from build123d import *

# Parameters (mm, degrees)
BOSS_EXTRUDE1_DEPTH       = 4.7625
SKETCH2_R                 = 3.302
BOSS_EXTRUDE2_DEPTH       = 3.175
SKETCH3_W                 = 12.827
SKETCH3_H                 = 4.8768
SKETCH3_W_2               = 4.8768
SKETCH3_H_2               = 12.827
PANEL_SLOTS_DEPTH         = 5.7625
BOSS_EXTRUDE8_DEPTH       = 4.7625
F_6_CLEARANCE_HOLE2_D     = 3.7973
F_6_CLEARANCE_HOLE2_DEPTH = 25.4
F_6_CLEARANCE_HOLE2_TIP   = 1.140824014
BOSS_EXTRUDE9_DEPTH       = 4.7625
F_6_CLEARANCE_HOLE3_D     = 3.7973
F_6_CLEARANCE_HOLE3_DEPTH = 25.4
F_6_CLEARANCE_HOLE3_TIP   = 1.140824014
FILLET1_R                 = 2.54
FILLET2_R                 = 2.54


with BuildPart() as part:
    # Sketch1 → Boss-Extrude1 (new body)
    with BuildSketch(Plane.XY):
        Polygon((-150.669615327, -62.417005507), (-62.404018861, -150.674994572), (62.417005507, -150.669615327), (150.674994572, -62.404018861), (150.669615327, 62.417005507), (62.404018861, 150.674994572), (-62.417005507, 150.669615327), (-150.674994572, 62.404018861), align=None)
        Polygon((-137.969842044, -57.155945955), (-57.144053939, -137.974767879), (57.155945955, -137.969842044), (137.974767879, -57.144053939), (137.969842044, 57.155945955), (57.144053939, 137.974767879), (-57.155945955, 137.969842044), (-137.974767879, 57.144053939), align=None, mode=Mode.SUBTRACT)
    extrude(amount=BOSS_EXTRUDE1_DEPTH)

    # Sketch2 → Boss-Extrude2 (add)
    with BuildSketch(Plane.XY.offset(4.7625)):
        with BuildLine():
            Line((-104.300258744, 90.821465649), (-90.83045509, 104.292430334))
            ThreePointArc((-90.83045509, 104.292430334), (-90.829874575, 90.822046164), (-104.300258744, 90.821465649))
        make_face()
        with Locations((-94.197615746, 94.189497078)):
            Circle(SKETCH2_R, mode=Mode.SUBTRACT)
        with BuildLine():
            Line((104.292430334, 90.83045509), (90.821465649, 104.300258744))
            ThreePointArc((90.821465649, 104.300258744), (90.822046164, 90.829874575), (104.292430334, 90.83045509))
        make_face()
        with Locations((94.189497078, 94.197615746)):
            Circle(SKETCH2_R, mode=Mode.SUBTRACT)
        with BuildLine():
            Line((104.300258744, -90.821465649), (90.83045509, -104.292430334))
            ThreePointArc((90.83045509, -104.292430334), (90.829874575, -90.822046164), (104.300258744, -90.821465649))
        make_face()
        with Locations((94.197615746, -94.189497078)):
            Circle(SKETCH2_R, mode=Mode.SUBTRACT)
        with BuildLine():
            Line((-104.292430334, -90.83045509), (-90.821465649, -104.300258744))
            ThreePointArc((-90.821465649, -104.300258744), (-90.822046164, -90.829874575), (-104.292430334, -90.83045509))
        make_face()
        with Locations((-94.189497078, -94.197615746)):
            Circle(SKETCH2_R, mode=Mode.SUBTRACT)
    extrude(amount=-BOSS_EXTRUDE2_DEPTH)

    # Sketch3 → Panel Slots (cut, through all)
    with BuildSketch(Plane.XY.offset(4.7625)):
        with Locations((-38.105945973, 145.908163017)):
            Rectangle(SKETCH3_W, SKETCH3_H)
        with Locations((12.69405398, 145.910352276)):
            Rectangle(SKETCH3_W, SKETCH3_H)
        Polygon((82.486917215, 127.306804135), (73.416858533, 136.376862817), (69.968440182, 132.928444466), (79.038498864, 123.858385784), align=None)
        Polygon((114.961071356, 87.938909374), (105.891012674, 97.008968056), (109.339431024, 100.457386406), (118.409489706, 91.387327724), align=None)
        with Locations((145.908163017, 38.105945973)):
            Rectangle(SKETCH3_W_2, SKETCH3_H_2)
        with Locations((145.910352276, -12.69405398)):
            Rectangle(SKETCH3_W_2, SKETCH3_H_2)
        Polygon((127.306804135, -82.486917215), (136.376862817, -73.416858533), (132.928444466, -69.968440182), (123.858385784, -79.038498864), align=None)
        Polygon((87.938909374, -114.961071356), (97.008968056, -105.891012674), (100.457386406, -109.339431024), (91.387327724, -118.409489706), align=None)
        with Locations((38.105945973, -145.908163017)):
            Rectangle(SKETCH3_W, SKETCH3_H)
        with Locations((-12.69405398, -145.910352276)):
            Rectangle(SKETCH3_W, SKETCH3_H)
        Polygon((-82.486917215, -127.306804135), (-73.416858533, -136.376862817), (-69.968440182, -132.928444466), (-79.038498864, -123.858385784), align=None)
        Polygon((-114.961071356, -87.938909374), (-105.891012674, -97.008968056), (-109.339431024, -100.457386406), (-118.409489706, -91.387327724), align=None)
        with Locations((-145.908163017, -38.105945973)):
            Rectangle(SKETCH3_W_2, SKETCH3_H_2)
        with Locations((-145.910352276, 12.69405398)):
            Rectangle(SKETCH3_W_2, SKETCH3_H_2)
        Polygon((-127.306804135, 82.486917215), (-136.376862817, 73.416858533), (-132.928444466, 69.968440182), (-123.858385784, 79.038498864), align=None)
        Polygon((-87.938909374, 114.961071356), (-97.008968056, 105.891012674), (-100.457386406, 109.339431024), (-91.387327724, 118.409489706), align=None)
    extrude(amount=-PANEL_SLOTS_DEPTH, mode=Mode.SUBTRACT)

    # Sketch9 → Boss-Extrude8 (add)
    with BuildSketch(Plane.XY.offset(4.7625)):
        with BuildLine():
            Line((-62.417005507, 150.669615327), (-43.367005525, 150.6704363))
            ThreePointArc((-43.367005525, 150.6704363), (-52.892416003, 160.195025805), (-62.417005507, 150.669615327))
        make_face()
        with BuildLine():
            Line((62.404018861, 150.674994572), (43.354018879, 150.6741736))
            ThreePointArc((43.354018879, 150.6741736), (52.878608384, 160.199584077), (62.404018861, 150.674994572))
        make_face()
        with BuildLine():
            Line((62.417005507, -150.669615327), (43.367005525, -150.6704363))
            ThreePointArc((43.367005525, -150.6704363), (52.892416003, -160.195025805), (62.417005507, -150.669615327))
        make_face()
        with BuildLine():
            Line((-62.404018861, -150.674994572), (-43.354018879, -150.6741736))
            ThreePointArc((-43.354018879, -150.6741736), (-52.878608384, -160.199584077), (-62.404018861, -150.674994572))
        make_face()
    extrude(amount=-BOSS_EXTRUDE8_DEPTH)

    # #6 Clearance Hole2
    with Locations(Plane.XY.offset(4.7625)):
        with Locations((-53.18125, 152.4), (53.18125, 152.4), (53.18125, -152.4), (-53.18125, -152.4), (0, 0)):
            Hole(F_6_CLEARANCE_HOLE2_D / 2, depth=F_6_CLEARANCE_HOLE2_DEPTH)
            with Locations((0, 0, -(F_6_CLEARANCE_HOLE2_DEPTH + F_6_CLEARANCE_HOLE2_TIP / 2))):  # 118° drill point
                Cone(0, F_6_CLEARANCE_HOLE2_D / 2, F_6_CLEARANCE_HOLE2_TIP, mode=Mode.SUBTRACT)

    # Sketch13 → Boss-Extrude9 (add)
    with BuildSketch(Plane.XY.offset(4.7625)):
        with BuildLine():
            Line((137.205190918, -75.874983545), (150.674994572, -62.404018861))
            Line((150.674994572, -62.404018861), (150.6741736, -43.354018879))
            ThreePointArc((150.6741736, -43.354018879), (168.275213823, -69.693379761), (137.205190918, -75.874983545))
        make_face()
        with BuildLine():
            Line((137.198650643, 75.886809161), (150.669615327, 62.417005507))
            Line((150.669615327, 62.417005507), (150.6704363, 43.367005525))
            ThreePointArc((150.6704363, 43.367005525), (168.269206233, 69.707883367), (137.198650643, 75.886809161))
        make_face()
        with BuildLine():
            Line((-150.674994581, 62.404018861), (-150.674173609, 43.354018879))
            ThreePointArc((-150.674173609, 43.354018879), (-168.275213832, 69.693379761), (-137.205190927, 75.874983545))
            Line((-137.205190927, 75.874983545), (-150.674994581, 62.404018861))
        make_face()
        with BuildLine():
            Line((-150.669615336, -62.417005507), (-150.670436308, -43.367005525))
            ThreePointArc((-150.670436308, -43.367005525), (-168.269206241, -69.707883367), (-137.198650652, -75.886809161))
            Line((-137.198650652, -75.886809161), (-150.669615336, -62.417005507))
        make_face()
    extrude(amount=-BOSS_EXTRUDE9_DEPTH)

    # #6 Clearance Hole3
    with Locations(Plane.XY.offset(4.7625)):
        with Locations((160.963744866, 66.681493332), (160.971633964, -66.668506668), (-160.963744823, -66.681493314), (-160.971634093, 66.668506686)):
            Hole(F_6_CLEARANCE_HOLE3_D / 2, depth=F_6_CLEARANCE_HOLE3_DEPTH)
            with Locations((0, 0, -(F_6_CLEARANCE_HOLE3_DEPTH + F_6_CLEARANCE_HOLE3_TIP / 2))):  # 118° drill point
                Cone(0, F_6_CLEARANCE_HOLE3_D / 2, F_6_CLEARANCE_HOLE3_TIP, mode=Mode.SUBTRACT)

    # Fillet1
    fillet1_edges = [part.edges().sort_by_distance(p)[0] for p in [
        (-62.417005507, 150.669615327, 2.38125),
        (62.404018861, 150.674994572, 2.38125),
        (62.417005507, -150.669615327, 2.38125),
        (-62.404018861, -150.674994572, 2.38125),
        (-43.367005525, 150.6704363, 2.38125),
        (43.354018879, 150.6741736, 2.38125),
        (43.367005525, -150.6704363, 2.38125),
        (-43.354018879, -150.6741736, 2.38125),
        (150.6704363, 43.367005525, 2.38125),
        (137.198650643, 75.886809161, 2.38125),
        (150.6741736, -43.354018879, 2.38125),
        (137.205190918, -75.874983545, 2.38125),
        (-137.198650652, -75.886809161, 2.38125),
        (-137.205190927, 75.874983545, 2.38125),
        (-150.674173609, 43.354018879, 2.38125),
    ]]
    fillet(fillet1_edges, radius=FILLET1_R)

    # Fillet2
    fillet2_edges = [part.edges().sort_by_distance(p)[0] for p in [
        (-90.83045509, 104.292430334, 3.175),
        (-104.300258744, 90.821465649, 3.175),
        (104.292430334, 90.83045509, 3.175),
        (90.821465649, 104.300258744, 3.175),
        (90.83045509, -104.292430334, 3.175),
        (104.300258744, -90.821465649, 3.175),
        (-104.292430334, -90.83045509, 3.175),
        (-90.821465649, -104.300258744, 3.175),
    ]]
    fillet(fillet2_edges, radius=FILLET2_R)


solid = part.part
Design review of the part built by this model. Coordinates are the model's own, in mm. A direction names the side the tool comes from. Round coordinates to 2 decimals unless told otherwise and drop trailing zeros. Write each loop counter-clockwise with the first axis right and the second up, starting at its lowest first coordinate (ties: lowest second). Pieces come first, ordered by that corner, then holes.
Item 1: Wall thickness on L1, parallel to Y at x = -15.5, z = 1.35; L2, parallel to X at y = 126, z = 1.7: over which ranges is each line inside the solid? List them lowest first.
Item 2: Consider section A-A on y = -49. Give the boundary of the cut face in (x, z), and give its area (3 significant figures).
Item 3: For faces 1 (the cylindrical face through (-53.26, -160.19, 2.41)), 2 (the flat face through (-110.5, -92.4, 2.4)), list the 3-axis set-ups (+Z, -Z, +X, -X, +Y, -Y) from which the entire face can be reached by the end or side of a thin tool; tool diameter is ignored.
Item 4: Draft analysis for pull direction X (two halves, no side actions). For faces 3 (the flat face through (-96.3, 97, 1.588)), 4 (the flat face through (78.015, 131.778, 2.415)), 5 (the flat face through (89, -94, 4.762)), state which applies: released by +X, released by -X, zero draft, split by the parting line, or undercut.
Item 5: Consider section B-B on z = 2.45. Count the separate pieces of the cut face and the enclosed holes in it, and give its area (3 significant figures).
Item 6: For pin 1 Ø2 at (y, z) = (123.5, 3) entering from +X; pin 2 Ø1.4 at (y, z) = (-7.5, 1.5) entering from +X; pin 3 Ø1.4 at (x, z) = (146, 1.5) entering from -Y, all flat-tipped, find the tip position at first contact; note any pin that passes through.
Check values:
1. L1: y = -150.67 to -148.35, -143.47 to -137.97, 137.97 to 150.67
1. L2: x = -87.08 to -69.12, 69.12 to 76.9, 81.18 to 87.08
2. outline: (-164.19, 0) - (-137.97, 0) - (-137.97, 4.76) - (-164.19, 4.76) - close; (137.97, 0) - (164.21, 0) - (164.21, 4.76) - (137.97, 4.76) - close
2. area: 250 mm2
3. face 1: +Z, -Z, -Y
3. face 2: +Z, -Z
4. face 3: undercut
4. face 4: undercut
4. face 5: zero draft
5. separate pieces: 1
5. enclosed holes: 29
5. area: 14,900 mm2
6. pin 1: stops at x = 90.58
6. pin 2: stops at x = 150.67
6. pin 3: stops at y = -81.03
